Part print with two shaded views. Sizes in mm from the minimum x, y, z corner. A direction names the side the tool comes from. Coordinates: 2 decimals unless noted, no trailing zeros. Loops run counter-clockwise (first coordinate to the right, second up) from the corner with the lowest first, then second, coordinate; pieces in that order, holes last. Notation, with made-up numbers: (8, 61.5) -> (21, 61.5) arc R20 cw to (21, 65.5) -> close; hole circle Ø11 at (-32, 12.5). An arc over 180 degrees is marked (long way). One line per item, written item: value. Start each with the question number.
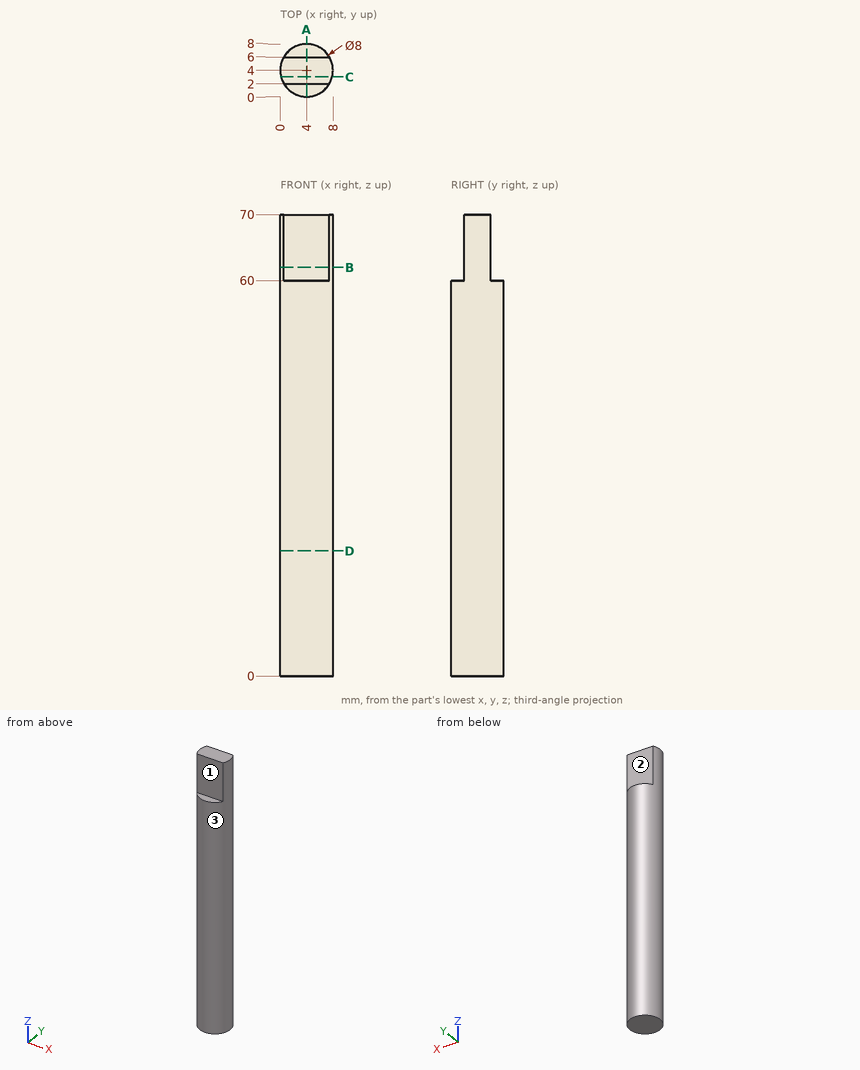
Item 1: Probe probe 1 along Y at (x, z) = (4.25, 29.5); probe 2 along X at (y, z) = (7.5, 14.5). List the from-to ranges inside material, lowest first.
Item 2: Band-saw the part on A-A, the plane x = 4. List the corners of the cut face in (y, z).
Item 3: Tool access for the marked faces 1, 2 and 3: list every direction of +Z, -Z, +X, -X, +Y, -Y with a clear straight run to the whole face (end or side of a thin tool).
Item 4: Band-saw the part on C-C, the plane y = 3. List the corners of the cut face in (x, z), and give its area (3 significant figures).
Item 5: Band-saw the part on D-D, the plane z = 19. List the corners of the cut face in (x, y).
Item 6: Band-saw the part on B-B, the plane z = 62. List the corners of the cut face in (x, y).
Item 7: Drop flat-ended pins along their axis: pin 1 Ø1.5 at (y, z) = (6.5, 42) entering from +X; pin 2 Ø1.5 at (x, z) = (1, 9.5) entering from -Y; pin 3 Ø2 at (x, z) = (3.5, 65) entering from -Y. Give the stop position or say it passes through.
Worked out:
1. probe 1: y = 0.01 to 7.99
1. probe 2: x = 2.06 to 5.94
2. outline: (0, 0) -> (8, 0) -> (8, 60) -> (6, 60) -> (6, 70) -> (2, 70) -> (2, 60) -> (0, 60) -> close
3. face 1: +Z, +X, -X, -Y
3. face 2: +Z, +X, -X, +Y
3. face 3: +Z, -Z
4. outline: (0.13, 0) -> (7.87, 0) -> (7.87, 70) -> (0.13, 70) -> close
4. area: 542 mm²
5. outline: circle Ø8 at (4, 4)
6. outline: (0.54, 2) -> (7.46, 2) arc R4 ccw to (7.46, 6) -> (0.54, 6) arc R4 ccw to start
7. pin 1: stops at x = 7.6
7. pin 2: stops at y = 0.69
7. pin 3: stops at y = 2
